```python
from build123d import *

# Parameters (mm, degrees)
F1_DEPTH       = 12.5
F3_D           = 3
F3_CBORE_D     = 5
F3_CBORE_DEPTH = 1.5
F4_DEPTH       = 4
F5_DEPTH       = 4.5
F7_W           = 52.7206266809
F7_H           = 3
F8_DEPTH       = 2
F10_DEPTH      = 2
F12_D          = 1
F12_DEPTH      = 3.5
F12_TIP        = 0.3004303095


with BuildPart() as f1:
    # F0 (on Top) → F1 (new body, symmetric)
    with BuildSketch(Plane.XY):
        with BuildLine():
            Line((-6.5277831331, -11.7825440413), (-8.5277831331, -11.7825440413))
            ThreePointArc((-8.5277831331, -11.7825440413), (-9.2348899143, -12.0754372601), (-9.5277831331, -12.7825440413))
            Line((-9.5277831331, -12.7825440413), (-9.5277831331, -14.7825440413))
            Line((-9.5277831331, -14.7825440413), (-2.5277831331, -14.7825440413))
            ThreePointArc((-2.5277831331, -14.7825440413), (-2.2348899143, -14.0754372601), (-1.5277831331, -13.7825440413))
            Line((-1.5277831331, -13.7825440413), (-1.0277831331, -13.7825440413))
            ThreePointArc((-1.0277831331, -13.7825440413), (1.4470906011, -14.8076703072), (2.4722168669, -17.2825440413))
            Line((2.4722168669, -17.2825440413), (2.4722168669, -31.7825440413))
            Line((2.4722168669, -31.7825440413), (4.4722168669, -31.7825440413))
            ThreePointArc((4.4722168669, -31.7825440413), (5.1793236481, -31.4896508225), (5.4722168669, -30.7825440413))
            Line((5.4722168669, -30.7825440413), (5.4722168669, -12.7825440413))
            ThreePointArc((5.4722168669, -12.7825440413), (5.1793236481, -12.0754372601), (4.4722168669, -11.7825440413))
            Line((4.4722168669, -11.7825440413), (1.472, -11.7825440413))
            Line((1.472, -11.7825440413), (-6.5277831331, -11.7825440413))
        make_face()
    extrude(amount=F1_DEPTH, both=True)

    # F3 (through all)
    with Locations(Plane.YZ.offset(5.4722168669)):
        with Locations((-25.7825440413, 7.5), (-25.7825440413, -7.5)):
            CounterBoreHole(F3_D / 2, F3_CBORE_D / 2, F3_CBORE_DEPTH)

    # F0 (on Top) → F4 (join, symmetric)
    with BuildSketch(Plane.XY):
        with BuildLine():
            Line((-6.528, -0.9138678433), (-8.5277831331, -11.7825440413))
            Line((-8.5277831331, -11.7825440413), (-6.5277831331, -11.7825440413))
            Line((-6.5277831331, -11.7825440413), (1.472, -11.7825440413))
            Line((1.472, -11.7825440413), (1.472, 35.2174559587))
            ThreePointArc((1.472, 35.2174559587), (-0.2919320225, 33.7453200037), (-2.528, 33.2174559587))
            Line((-2.528, 33.2174559587), (-2.528, 23.2174559587))
            Line((-2.528, 23.2174559587), (-6.528, 23.2174559587))
            Line((-6.528, 23.2174559587), (-6.528, -0.9138678433))
        make_face()
    extrude(amount=F4_DEPTH, both=True)

    # F0 (on Top) → F5 (join, symmetric)
    with BuildSketch(Plane.XY):
        with BuildLine():
            ThreePointArc((-2.528, 33.2174559587), (-0.2919320225, 33.7453200037), (1.472, 35.2174559587))
            ThreePointArc((1.472, 35.2174559587), (1.944135955, 40.4535239362), (-2.528, 43.2174559587))
            Line((-2.528, 43.2174559587), (-2.528, 41.2174559587))
            ThreePointArc((-2.528, 41.2174559587), (0.472, 38.2174559587), (-2.528, 35.2174559587))
            Line((-2.528, 35.2174559587), (-2.528, 33.2174559587))
        make_face()
    extrude(amount=F5_DEPTH, both=True)

    # F7 (on offset) → F8 (cut, symmetric)
    with BuildSketch(Plane.YZ.offset(-2.528)):
        with Locations((10.1688103074, 0)):
            Rectangle(F7_W, F7_H)
    extrude(amount=F8_DEPTH, both=True, mode=Mode.SUBTRACT)

    # F9 (on Top) → F10 (cut, symmetric)
    with BuildSketch(Plane.XY):
        Polygon((-1.2336979853, -0.9498164291), (-4.6429014765, -0.9498164291), (-7.5818696059, -16.5851321071), (-1.2336979853, -16.5851321071), align=None)
    extrude(amount=F10_DEPTH, both=True, mode=Mode.SUBTRACT)

    # F12
    with Locations(Plane(origin=(-2.528, 0, 0), x_dir=(0, -1, 0), z_dir=(-1, 0, 0))):
        with Locations((-28.2174559587, -2.5), (-28.2174559587, 2.5)):
            Hole(F12_D / 2, depth=F12_DEPTH)
            with Locations((0, 0, -(F12_DEPTH + F12_TIP / 2))):  # 118° drill point
                Cone(0, F12_D / 2, F12_TIP, mode=Mode.SUBTRACT)


solid = f1.part
```
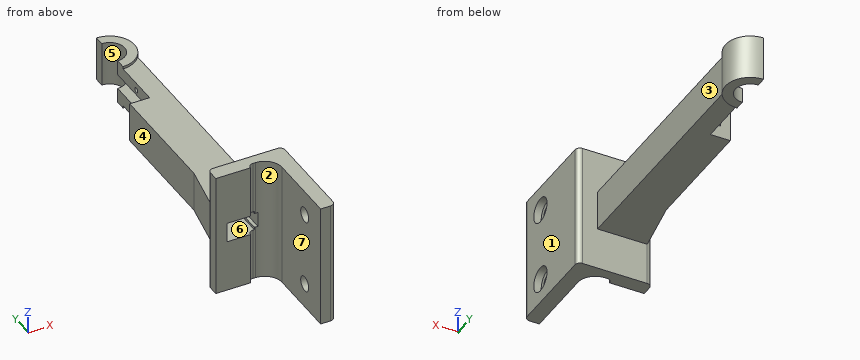
CAD build for the part. Positions are in the model's coordinates, mm. Face numbers are marked on the shaded views. A direction names the side the tool comes from. Coordinates: 2 decimals unless noted, no trailing zeros. Write each loop counter-clockwise with the first axis right and the second up, starting at its lowest first coordinate (ties: lowest second). Pieces come first, ordered by that corner, then holes.
(1) Cut at D-D, the plane y = -18.5. List the corners of the cut face in (x, z), and give its area (3 significant figures).
(2) 3-axis set-ups, long thin cutter, end or side, ignore diameter. For the marked faces 4, 5, 6 and 7: which of +Z, -Z, +X, -X, +Y, -Y reach the whole face in a straight line?
(3) Two-plate mould, pull along Y, no slides. Class the marked faces 1, 2 and 3: +Y half, -Y half, draft (parallel to the pull), parting line (faces both ways), or undercut.
(4) Cut at B-B, the plane y = 20.5. List the corners of the cut face in (x, z), and give its area (3 significant figures).
(5) Drill centre lines: probe 1 along Y at (x, z) = (-0.9, 2.5) (3 decimals); probe 2 along Y at (x, z) = (-1.1, 2.5); probe 3 along X at (y, z) = (7.5, -1.75). Where is each one in solid material? Low to high.
(6) Cut at C-C, the plane z = -11. List the corners of the cut face in (x, y).
(7) Cut at A-A, the plane z = -7.5. List the corners of the cut face in (x, y).
(8) Flat gauge pins, fed straight in: pin 1 (3.5 mm diameter, centred on y = 7, z = 0.5, fed in from -X); pin 2 (2.5 mm diameter, centred on y = -25.78, z = 7.5, fed in from +X); pin 3 (2.5 mm diameter, centred on y = 31, z = -3, fed in from -X); pin 4 (3 mm diameter, centred on x = -6, y = 16.5, fed in from +Z). Where does each tip first touch, or does it go through?
Geometry says:
1. outline: (2.47, -12.5) - (5.47, -12.5) - (5.47, 12.5) - (2.47, 12.5) - close
1. area: 75.0 mm2
2. face 4: +Z, -Z, -X, +Y
2. face 5: +Z, -Z, -X
2. face 6: -Y
2. face 7: +Z, -Z, -X, -Y
3. face 1: draft
3. face 2: -Y half
3. face 3: undercut
4. outline: (-6.53, -4) - (1.47, -4) - (1.47, 4) - (-6.53, 4) - close; hole (-4.53, -1.5) - (-0.53, -1.5) - (-0.53, 1.5) - (-4.53, 1.5) - close
4. area: 52.0 mm2
5. probe 1: y = -13.785 to 27.717, 28.717 to 35.698, 40.737 to 42.945
5. probe 2: y = -13.78 to 27.72, 28.72 to 35.58, 40.86 to 43.01
5. probe 3: x = -6.53 to 1.47
6. outline: (-9.53, -14.78) - (-2.53, -14.78) arc R1 cw to (-1.53, -13.78) - (-1.03, -13.78) arc R3.5 cw to (2.47, -17.28) - (2.47, -31.78) - (4.47, -31.78) arc R1 ccw to (5.47, -30.78) - (5.47, -12.78) arc R1 ccw to (4.47, -11.78) - (-8.53, -11.78) arc R1 ccw to (-9.53, -12.78) - close
7. outline: (-9.53, -14.78) - (-2.53, -14.78) arc R1 cw to (-1.53, -13.78) - (-1.03, -13.78) arc R3.5 cw to (2.47, -17.28) - (2.47, -24.28) - (3.97, -24.28) - (3.97, -23.28) - (5.47, -23.28) - (5.47, -12.78) arc R1 ccw to (4.47, -11.78) - (-8.53, -11.78) arc R1 ccw to (-9.53, -12.78) - close; (2.47, -31.78) - (4.47, -31.78) arc R1 ccw to (5.47, -30.78) - (5.47, -28.28) - (3.97, -28.28) - (3.97, -27.28) - (2.47, -27.28) - close
8. pin 1: stops at x = -6.53
8. pin 2: passes through
8. pin 3: stops at x = -2.53
8. pin 4: stops at z = 4
